For this review, take the finished solid that the model builds, in its own axes (mm). A direction names the side the tool comes from. Coordinates: 2 decimals unless noted, no trailing zeros. Order: outer loops, then holes, each group sorted by start corner. A loop starts at its lowest first (then second) coordinate and runs counter-clockwise, first axis right, second up.
from build123d import *

# Parameters (mm, degrees)
SALIENTE_EXTRUIR1_DEPTH    = 2.4
CROQUIS2_R                 = 6.86
SALIENTE_EXTRUIR2_DEPTH    = 10
CROQUIS3_W                 = 8
CROQUIS3_H                 = 8
CORTAR_EXTRUIR1_DEPTH      = 8
CORTAR_EXTRUIR2_DEPTH      = 20.431513065
CORTAR_EXTRUIR2_DEPTH_BACK = 20.431513065
CROQUIS5_R                 = 2


with BuildPart() as part:
    # Croquis1 → Saliente-Extruir1 (new body)
    with BuildSketch(Plane(origin=(0, 0, 0), x_dir=(1, 0, 0), z_dir=(0, 1, 0))):
        with BuildLine():
            Line((-6.008085542, 3.310967853), (-2.306310946, 10.028211696))
            ThreePointArc((-2.306310946, 10.028211696), (0, 10.29), (2.306310946, 10.028211696))
            Line((2.306310946, 10.028211696), (6.008085542, 3.310967853))
            ThreePointArc((6.008085542, 3.310967853), (6.86, 0), (6.008085542, -3.310967853))
            Line((6.008085542, -3.310967853), (2.306310946, -10.028211696))
            ThreePointArc((2.306310946, -10.028211696), (0, -10.29), (-2.306310946, -10.028211696))
            Line((-2.306310946, -10.028211696), (-6.008085542, -3.310967853))
            ThreePointArc((-6.008085542, -3.310967853), (-6.86, 0), (-6.008085542, 3.310967853))
        make_face()
    extrude(amount=SALIENTE_EXTRUIR1_DEPTH)

    # Croquis2 → Saliente-Extruir2 (add)
    with BuildSketch(Plane(origin=(0, 2.4, 0), x_dir=(1, 0, 0), z_dir=(0, 1, 0))):
        with Locations(Location((0, 0, 0), (0, 0, 28.858514896))):
            Circle(CROQUIS2_R)
    extrude(amount=SALIENTE_EXTRUIR2_DEPTH)

    # Croquis3 → Cortar-Extruir1 (cut)
    with BuildSketch(Plane(origin=(0, 12.4, 0), x_dir=(1, 0, 0), z_dir=(0, 1, 0))):
        Rectangle(CROQUIS3_W, CROQUIS3_H)
    extrude(amount=-CORTAR_EXTRUIR1_DEPTH, mode=Mode.SUBTRACT)

    # Croquis5 → Cortar-Extruir2 (cut, two sides: drawn at the far end of the back side and taken through both)
    with BuildSketch(Plane(origin=(-4, 0, 0), x_dir=(0, 0, -1), z_dir=(1, 0, 0)).offset(-CORTAR_EXTRUIR2_DEPTH_BACK)):
        with Locations(Location((0, 8.4, 0), (0, 0, 270))):
            Circle(CROQUIS5_R)
    extrude(amount=CORTAR_EXTRUIR2_DEPTH + CORTAR_EXTRUIR2_DEPTH_BACK, mode=Mode.SUBTRACT)


solid = part.part
1. Take a section at B-B, the plane y = 7.75. Give the boundary of the cut face in (x, z), plus the area to 3 significant figures.
Answer below:
outline: (-6.59, -1.89) arc R6.86 ccw to (6.59, -1.89) - (4, -1.89) - (4, -4) - (-4, -4) - (-4, -1.89) - close; (-6.59, 1.89) - (-4, 1.89) - (-4, 4) - (4, 4) - (4, 1.89) - (6.59, 1.89) arc R6.86 ccw to start
area: 62.9 mm2
2. Take a section at A-A, the plane z = 0. Give the boundary of the cut face in (x, y).
Answer below:
outline: (-6.86, 0) - (6.86, 0) - (6.86, 6.4) - (4, 6.4) - (4, 4.4) - (-4, 4.4) - (-4, 6.4) - (-6.86, 6.4) - close; (-6.86, 10.4) - (-4, 10.4) - (-4, 12.4) - (-6.86, 12.4) - close; (4, 10.4) - (6.86, 10.4) - (6.86, 12.4) - (4, 12.4) - close
3. Clearance check with flat-ended pins moving along their axes: pin 1 Ø1.5 at (x, y) = (-1, 5.5) entering from -Z; pin 2 Ø1.5 at (y, z) = (7, -2.5) entering from +X; pin 3 Ø2.5 at (y, z) = (8.5, 0) entering from -X; pin 4 Ø1 at (y, z) = (9, 5) entering from +X. State where each tip first meets the part, or that it passes through.
Answer below:
pin 1: stops at z = -6.86
pin 2: stops at x = 6.63
pin 3: passes through
pin 4: stops at x = 5.18
4. Machinability: for faces 5 (the face through (1.1, 12.4, -4.2)), 6 (the face through (0, 4.4, 0)), which of the approach directions +Z, -Z, +X, -X, +Y, -Y give a long, thin tool a straight path to every point of the face, cutting with its end or side? Answer none if there is none.
Answer below:
face 5: +Z, -Z, +X, -X, +Y
face 6: +Y
5. The part is to be moulded in two halves that separate along Z. For faces 1 (the face through (0, 2.4, -8)), 2 (the face through (-4.13, 1.18, 6.72)), 3 (the face through (-4.183, 1.183, -6.623)), 4 (the face through (0, 8, -4)), say which applies: +Z half, -Z half, draft (parallel to the pull), parting line (faces both ways), or undercut.
Answer below:
face 1: draft
face 2: +Z half
face 3: -Z half
face 4: undercut
6. Take a section at C-C, the plane x = 4.5. Give the boundary of the cut face in (y, z).
Answer below:
outline: (0, -6.05) - (2.4, -6.05) - (2.4, -5.18) - (12.4, -5.18) - (12.4, 5.18) - (2.4, 5.18) - (2.4, 6.05) - (0, 6.05) - close; hole circle Ø4 at (8.4, 0)
7. Take a section at D-D, the plane x = 0. Give the boundary of the cut face in (y, z), plus the area to 3 significant figures.
Answer below:
outline: (0, -10.29) - (2.4, -10.29) - (2.4, -6.86) - (12.4, -6.86) - (12.4, -4) - (4.4, -4) - (4.4, 4) - (12.4, 4) - (12.4, 6.86) - (2.4, 6.86) - (2.4, 10.29) - (0, 10.29) - close
area: 123 mm2
8. To check wall thickness, follow L1, parallel to X at y = 11, z = 0; L2, parallel to Y at x = -1.5, z = 6.75; L3, parallel to Z at x = 5.15, y = 8.4. State the ranges of each line that lie inside material, in increasing order.
Answer below:
L1: x = -6.86 to -4, 4 to 6.86
L2: y = 0 to 2.4
L3: z = -4.53 to -2, 2 to 4.53
